```python
from build123d import *

# Parameters (mm, degrees)
PAD_DEPTH       = 7.5
SKETCH001_W     = 157
SKETCH001_H     = 166.73666
POCKET_DEPTH    = 8
CHAMFER_SIZE    = 7.99
SKETCH002_R     = 4.9
PAD001_DEPTH    = 20
CHAMFER001_SIZE = 1
FILLET_R        = 3
SKETCH003_W     = 160
SKETCH003_H     = 1
POCKET001_DEPTH = 171


with BuildPart() as part:
    # Sketch → Pad (new body, symmetric)
    with BuildSketch(Plane.XZ):
        with BuildLine():
            Line((-90, 89.73666), (-90, -90))
            Line((-90, -90), (90, -90))
            Line((90, -90), (90, 89.73666))
            ThreePointArc((90, 89.73666), (87.071068, 96.807727), (80, 99.73666))
            Line((80, 99.73666), (-80, 99.73666))
            ThreePointArc((-80, 99.73666), (-87.071068, 96.807727), (-90, 89.73666))
        make_face()
    extrude(amount=PAD_DEPTH, both=True)

    # Sketch001 (on Face8 of Pad) → Pocket (cut)
    with BuildSketch(Plane.XZ.offset(7.5)):
        with Locations((0, 4.86833)):
            Rectangle(SKETCH001_W, SKETCH001_H)
    extrude(amount=-POCKET_DEPTH, mode=Mode.SUBTRACT)

    # Chamfer
    chamfer_edges = [part.edges().sort_by_distance(p)[0] for p in [
        (0, 0.5, 88.23666),
        (-78.5, 0.5, 4.86833),
        (0, 0.5, -78.5),
        (78.5, 0.5, 4.86833),
    ]]
    chamfer(chamfer_edges, length=CHAMFER_SIZE)

    # Sketch002 (on Face3 of Pocket) → Pad001 (join)
    with BuildSketch(Plane(origin=(0, 0, -90), x_dir=(1, 0, 0), z_dir=(0, 0, -1))):
        with Locations((-45, 0)):
            Circle(SKETCH002_R)
        with Locations((45, 0)):
            Circle(SKETCH002_R)
    extrude(amount=PAD001_DEPTH)

    # Chamfer001
    chamfer001_edges = [part.edges().sort_by_distance(p)[0] for p in [
        (40.1, 0, -90),
        (-49.9, 0, -90),
        (-49.9, 0, -110),
        (40.1, 0, -110),
    ]]
    chamfer(chamfer001_edges, length=CHAMFER001_SIZE)

    # Fillet
    fillet_edges = [part.edges().sort_by_distance(p)[0] for p in [
        (90, -7.5, -0.13167),
        (90, 7.5, -0.13167),
    ]]
    fillet(fillet_edges, radius=FILLET_R)

    # Sketch003 (on Face26 of Fillet) → Pocket001 (cut)
    with BuildSketch(Plane(origin=(0, 0, 99.73666), x_dir=(-1, 0, 0), z_dir=(0, 0, 1))):
        Rectangle(SKETCH003_W, SKETCH003_H)
    extrude(amount=-POCKET001_DEPTH, mode=Mode.SUBTRACT)


solid = part.part
```
Build history of the part. All positions in model axes, mm. A direction names the side the tool comes from. Give positions to 0.01 mm unless a question says otherwise; leave off trailing zeros. Write item = value, one per line. Start each with the question number.
(1) Which spindle directions (+Z, -Z, +X, -X, +Y, -Y) get a long thin tool onto all of the face, cutting with end or side? Do faces 5 (the cylindrical face through (40.105, -0.215, -99.874)), 6 (the flat face through (-1.099, -3.946, 84.693)), 7 (the flat face through (1, 0.5, 15)). Say none if no direction does.
(2) Pin check, flat tips, straight feed: pin 1 Ø3 at (x, z) = (-23.5, 69.5) entering from -Y; pin 2 Ø0.5 at (x, y) = (-21.5, 0) entering from +Z; pin 3 Ø1.5 at (x, y) = (-29, 0.5) entering from -Z. Stop position of each tip, or through.
(3) Probe L1, parallel to X at y = 0.25, z = 20.5; L2, parallel to Z at x = -14, y = 3.5; L3, parallel to Y at x = 47, z = 2. List the from-to ranges inside material, lowest first. Write a range as [from, to].
(4) Two-plate mould, pull along Y, no slides. Class faces 1 (the cylindrical face through (87.15, -0.06, 96.73)), 2 (the flat face through (0, -0.5, 84)), 3 (the cylindrical face through (-49.895, -0.215, -99.874)), 4 (the flat face through (-1, 7.5, 5)): released by +Y, released by -Y, zero draft, split by the parting line, or undercut.
Responses:
q1.face_5 = -Z
q1.face_6 = -Y
q1.face_7 = +Z
q2.pin_1 = 0.5
q2.pin_2 = -71.26
q2.pin_3 = -90
q3.L1 = [-90, -80], [80, 90]
q3.L2 = [-90, 99.74]
q3.L3 = [0.5, 7.5]
q4.face_1 = zero draft
q4.face_2 = undercut
q4.face_3 = split by the parting line
q4.face_4 = released by +Y
